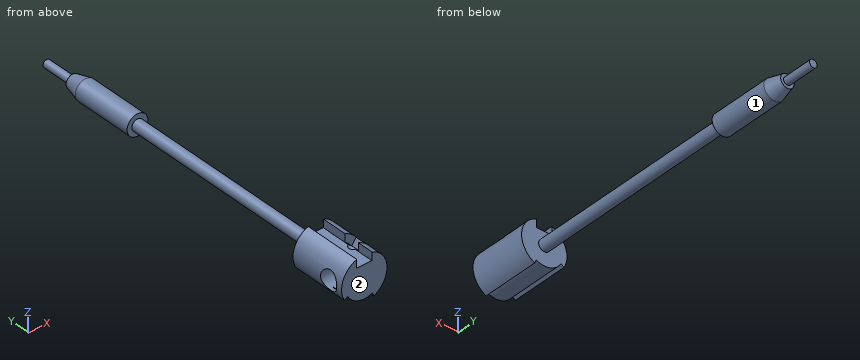
```python
from build123d import *

# Parameters (mm, degrees)
F0_R      = 1
F1_DEPTH  = 8
F2_R      = 2.75
F3_DEPTH  = 80
F4_SIZE2  = 1
F4_SIZE   = 4
F5_R      = 6
F5_R_2    = 2.75
F6_DEPTH  = 5
F7_DEPTH  = 10
F12_R     = 2.75
F12_R_2   = 1.5
F13_DEPTH = 55
F15_D     = 5
F15_DEPTH = 7
F15_START = 0.545644
F15_TIP   = 1.5021515476
F16_W     = 4
F16_H     = 15
F17_DEPTH = 2.5
F19_W     = 4.1
F19_H     = 2.1568542495
F20_ANGLE = 35
F28_DEPTH = 15


with BuildPart() as f1:
    # F0 (on Front) → F1 (new body)
    with BuildSketch(Plane.XZ):
        Circle(F0_R)
    extrude(amount=-F1_DEPTH)

    # F2 (on face) → F3 (join)
    with BuildSketch(Plane.XZ):
        Circle(F2_R)
    extrude(amount=F3_DEPTH)

    # F4
    f4_edges = [f1.edges().sort_by_distance(p)[0] for p in [
        (-2.75, 0, 0),
    ]]
    f4_side = f1.faces().sort_by_distance((-2.75, -40, 0))[0]
    chamfer(f4_edges, length=F4_SIZE, length2=F4_SIZE2, reference=f4_side)

    # F5 (on face) → F6 (join)
    with BuildSketch(Plane.XZ.offset(80)):
        Circle(F5_R)
        Circle(F5_R_2, mode=Mode.SUBTRACT)
    extrude(amount=-F6_DEPTH)

    # F7 (add): a face of the model
    f7_faces = [f1.faces().sort_by_distance(p)[0] for p in [
        (0, -80, 0),
    ]]
    extrude(f7_faces, amount=F7_DEPTH)

    # F12 (on face) → F13 (cut)
    with BuildSketch(Plane(origin=(0, -75, 0), x_dir=(-1, 0, 0), z_dir=(0, 1, 0))):
        Circle(F12_R)
        Circle(F12_R_2, mode=Mode.SUBTRACT)
    extrude(amount=F13_DEPTH, mode=Mode.SUBTRACT)

    # F15
    # its depths count from where the whole tool has entered the part; down to there all is cleared
    with Locations(Plane(origin=(-6, 0, 0), x_dir=(0, 1, 0), z_dir=(-1, 0, 0)).offset(-F15_START)):
        with Locations((-86, 0)):
            Hole(F15_D / 2, depth=F15_DEPTH)
            with Locations((0, 0, -(F15_DEPTH + F15_TIP / 2))):  # 118° drill point
                Cone(0, F15_D / 2, F15_TIP, mode=Mode.SUBTRACT)

    # F16 (on offset) → F17 (cut)
    with BuildSketch(Plane.XY.offset(6)):
        with Locations((0, -82.5)):
            Rectangle(F16_W, F16_H)
    extrude(amount=-F17_DEPTH, mode=Mode.SUBTRACT)

    # F19 (on face) → F20 (revolve, cut)
    with BuildSketch(Plane(origin=(2, 0, 0), x_dir=(0, -1, 0), z_dir=(-1, 0, 0))):
        with Locations((83.8, 4.5784271247)):
            Rectangle(F19_W, F19_H)
    revolve(axis=Axis((0, -80, 0), (0, 1, 0)), revolution_arc=F20_ANGLE, mode=Mode.SUBTRACT)

    # F25 (on face) → F26 (revolve, cut)
    with BuildSketch(Plane(origin=(-0.302441943, 0, 0.2117721284), x_dir=(0, -1, 0), z_dir=(-0.8191520443, 0, 0.5735764364))):
        with BuildLine():
            Line((83.8, 5.9141850277), (83.8, 3.4141850277))
            ThreePointArc((83.8, 3.4141850277), (85.05, 4.6641850277), (83.8, 5.9141850277))
        make_face()
    revolve(axis=Axis((2.3728246836, -83.8, 4.0324488288), (0.5735764364, 0, 0.8191520443)), mode=Mode.SUBTRACT)

    # F27 (on face) → F28 (cut)
    with BuildSketch(Plane.XZ.offset(90)):
        with BuildLine():
            ThreePointArc((-5.2477182428, -2.9088577215), (-1.8541019662, -5.7063390978), (2.5357095704, -5.4378467222))
            Line((2.5357095704, -5.4378467222), (2.1130913087, -4.5315389352))
            ThreePointArc((2.1130913087, -4.5315389352), (-1.5450849719, -4.7552825815), (-4.3730985357, -2.4240481012))
            Line((-4.3730985357, -2.4240481012), (-5.2477182428, -2.9088577215))
        make_face()
    extrude(amount=-F28_DEPTH, mode=Mode.SUBTRACT)


solid = f1.part
```
Input: part model. Units: mm. Frame: model coordinates. Face numbers are marked on the shaded views. A direction names the side the tool comes from. Give positions to 0.01 mm unless a question says otherwise; leave off trailing zeros. Loops run counter-clockwise (first coordinate to the right, second up) from the corner with the lowest first, then second, coordinate; pieces in that order, holes last.
1) Line query: L1, parallel to Z at x = -0.25, y = -86; L2, parallel to Z at x = -3.25, y = -86; L3, parallel to Y at x = 3.75, z = 0.25. Output: solid intervals per line, ascending.
A:
L1: z = -4.99 to -2.5, 2.5 to 3.5
L2: z = -3.8 to -2.5, 2.5 to 5.04
L3: y = -90 to -75
2) Contact query for flat-ended pins moving along their axis: pin 1 (1 mm diameter, centred on x = -1.5, z = -3, fed in from +Y); pin 2 (2.5 mm diameter, centred on y = -86, z = 4, fed in from +X); pin 3 (3 mm diameter, centred on x = 0.5, y = -84.5, fed in from +Z). Output: stop coordinate, or through.
A:
pin 1: stops at y = -75
pin 2: stops at x = 5.33
pin 3: stops at z = 3.5
3) Section query B-B on y = -71. Return the cut outline in (x, z), and give its area (3 significant figures).
A:
outline: circle Ø3 at (0, 0)
area: 7.07 mm2
4) Section query A-A on x = 0. Return the cut outline in (y, z), and give its area (3 significant figures).
A:
outline: (-90, -5) - (-75, -5) - (-75, -1.5) - (-20, -1.5) - (-20, -2.75) - (-4, -2.75) - (0, -1.75) - (0, -1) - (8, -1) - (8, 1) - (0, 1) - (0, 1.75) - (-4, 2.75) - (-20, 2.75) - (-20, 1.5) - (-75, 1.5) - (-75, 3.5) - (-90, 3.5) - close; hole circle Ø5 at (-86, 0)
area: 395 mm2
5) Reachability of the marked faces 1 and 2 from +Z, -Z, +X, -X, +Y, -Y: full face, straight path, thin tool, end or side. Return the list, or none.
A:
face 1: +Y
face 2: +Z, -Z, +X, -X, -Y
